from build123d import *

# Parameters (mm, degrees)
SKETCH1_R                = 12.446
BOSS_EXTRUDE1_DEPTH      = 25.4
BOSS_EXTRUDE1_DEPTH_BACK = 25.4
SKETCH2_R                = 3.5
BOSS_EXTRUDE2_DEPTH      = 2.54
SKETCH4_R                = 2
BOSS_EXTRUDE3_DEPTH      = 1.75
BOSS_EXTRUDE4_DEPTH      = 8
SKETCH6_R                = 1.5
CUT_EXTRUDE1_DEPTH       = 3.175
BOSS_EXTRUDE5_DEPTH      = 11.8364


with BuildPart() as part:
    # Sketch1 → Boss-Extrude1 (new body, two sides)
    with BuildSketch(Plane.XY) as boss_extrude1_sk:
        Circle(SKETCH1_R)
    extrude(amount=BOSS_EXTRUDE1_DEPTH)
    extrude(boss_extrude1_sk.sketch, amount=-BOSS_EXTRUDE1_DEPTH_BACK)

    # Sketch2 → Boss-Extrude2 (add)
    with BuildSketch(Plane.XY.offset(25.4)):
        Circle(SKETCH2_R)
    extrude(amount=BOSS_EXTRUDE2_DEPTH)

    # Sketch4 → Boss-Extrude3 (add)
    with BuildSketch(Plane.XY.offset(27.94)):
        Circle(SKETCH4_R)
    extrude(amount=BOSS_EXTRUDE3_DEPTH)

    # Sketch5 → Boss-Extrude4 (add)
    with BuildSketch(Plane.XY.offset(29.69)):
        with BuildLine():
            Line((1.405616757, 1.422758424), (-1.405616757, 1.422758424))
            ThreePointArc((-1.405616757, 1.422758424), (0, -2.081119268), (1.405616757, 1.422758424))
        make_face()
    extrude(amount=BOSS_EXTRUDE4_DEPTH)

    # Sketch6 → Cut-Extrude1 (cut)
    with BuildSketch(Plane.XY.offset(25.4)):
        with Locations((6.01040764, 6.01040764)):
            Circle(SKETCH6_R)
        with Locations((6.01040764, -6.01040764)):
            Circle(SKETCH6_R)
        with Locations((-6.01040764, -6.01040764)):
            Circle(SKETCH6_R)
        with Locations((-6.01040764, 6.01040764)):
            Circle(SKETCH6_R)
    extrude(amount=-CUT_EXTRUDE1_DEPTH, mode=Mode.SUBTRACT)

    # Sketch7 → Boss-Extrude5 (add)
    with BuildSketch(Plane(origin=(0, 0, -25.4), x_dir=(-1, 0, 0), z_dir=(0, 0, -1))):
        with BuildLine():
            Line((0, 12.446), (19.05, 12.446))
            Line((19.05, 12.446), (19.05, -12.446))
            Line((19.05, -12.446), (0, -12.446))
            ThreePointArc((0, -12.446), (-12.446, 0), (0, 12.446))
        make_face()
    extrude(amount=BOSS_EXTRUDE5_DEPTH)


solid = part.part
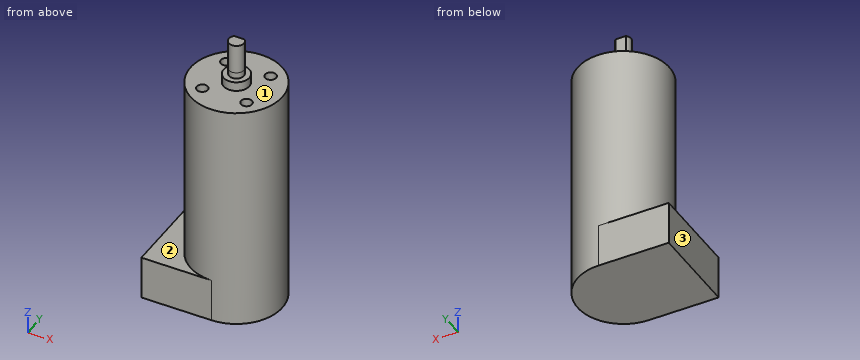
Source: CAD feature listing. Evaluate the final solid. Frame: model axes, mm. Face numbers are marked on the shaded views. A direction names the side the tool comes from. Round coordinates to 2 decimals unless told otherwise and drop trailing zeros. Order: outer loops, then holes, each group sorted by start corner. A loop starts at its lowest first (then second) coordinate and runs counter-clockwise, first axis right, second up. Notation, with made-up numbers: (61, 77.5) - (71, 77.5) arc R16 cw to (71, 104.5) - close; hole circle Ø4 at (-26, 54). An arc over 180 degrees is marked (long way). Use a Markdown table: item, result. Add a question column.
1. Section query A-A (x = -10). Return the cut outline in (y, z), then the cut area to 3 significant figures.
2. Section query C-C (z = 12.5). Return the cut outline in (x, y).
3. Section query D-D (x = -16.5). Return the cut outline in (y, z), then the cut area to 3 significant figures.
4. Set-up query: the marked faces 1, 2 and 3. Return all of +Z, -Z, +X, -X, +Y, -Y with unobstructed straight access to the full face (end or side cutting, diameter ignored); none if empty.
5. First-contact query: pin 1 (5 mm diameter, centred on y = -10, z = 11.5, fed in from +X); pin 2 (2.5 mm diameter, centred on x = -6.5, y = -5.5, fed in from +Z); pin 3 (1.5 mm diameter, centred on x = 6.5, y = -6, fed in from +Z) (3 decimals). Flat tips, straight axial feed; report the tip coordinate or a pass-through.
6. Section query B-B (y = -8.25). Return the cut outline in (x, z), then the cut area to 3 significant figures.
7. Line query: probe 1 along Z at (x, y) = (-3, -8.75); probe 2 along Z at (x, y) = (-15, -2.75); probe 3 along Y at (x, z) = (3, -0.5). Output: solid intervals per line, ascending.
Derived:
| question | item | result |
|---|---|---|
| 1 | outline | (-12.45, -37.24) - (12.45, -37.24) - (12.45, -25.4) - (7.41, -25.4) - (7.41, 25.4) - (-7.41, 25.4) - (-7.41, -25.4) - (-12.45, -25.4) - close |
| 1 | area | 1,050 mm2 |
| 2 | outline | circle Ø24.89 at (0, 0) |
| 3 | outline | (-12.45, -37.24) - (12.45, -37.24) - (12.45, -25.4) - (-12.45, -25.4) - close |
| 3 | area | 295 mm2 |
| 4 | face 1 | +Z |
| 4 | face 2 | +Z, -X |
| 4 | face 3 | +Z, -Z, -X, +Y, -Y |
| 5 | pin 1 | x = 9.93 |
| 5 | pin 2 | z = 25.4 |
| 5 | pin 3 | z = 22.225 |
| 6 | outline | (-19.05, -37.24) - (9.32, -37.24) - (9.32, 25.4) - (-9.32, 25.4) - (-9.32, -25.4) - (-19.05, -25.4) - close |
| 6 | area | 1,280 mm2 |
| 7 | probe 1 | -37.24 to 25.4 |
| 7 | probe 2 | -37.24 to -25.4 |
| 7 | probe 3 | -12.08 to 12.08 |
